Part model, mm, in its own coordinate system. Give positions to 0.01 mm unless a question says otherwise; leave off trailing zeros. Loops run counter-clockwise (first coordinate to the right, second up) from the corner with the lowest first, then second, coordinate; pieces in that order, holes last. Notation, with made-up numbers: M 28.25,78 L 83.25,78 A22 ccw 83.25,86 Z; hole C -24.5,42.25 d6. An arc over 180 degrees is marked long. Put each result on its own line as item: value. Start each with the question number.
```python
from build123d import *

# Parameters (mm, degrees)
BOSS_EXTRU_1_DEPTH = 100
CONG_1_R           = 30


with BuildPart() as part:
    # Esquisse1 → Boss.-Extru.1 (new body)
    with BuildSketch(Plane.XY):
        with BuildLine():
            Line((36.827299657, 30), (22.5, 30))
            ThreePointArc((22.5, 30), (33.541019662, 16.770509831), (37.5, 0))
            ThreePointArc((37.5, 0), (33.541019662, -16.770509831), (22.5, -30))
            Line((22.5, -30), (36.827299657, -30))
            ThreePointArc((36.827299657, -30), (44.752355992, -15.920949505), (47.5, 0))
            ThreePointArc((47.5, 0), (44.752355992, 15.920949505), (36.827299657, 30))
        make_face()
    extrude(amount=BOSS_EXTRU_1_DEPTH)

    # Congé1
    # the kernel refuses this fillet: 30 mm, written as the material it takes off along each edge
    with BuildSketch(Plane(origin=(111.827299657, 30, 100), x_dir=(0, 0, -1), z_dir=(-1, 0, 0))) as cong_1_piece_1:
        with BuildLine():
            CenterArc((CONG_1_R, CONG_1_R), CONG_1_R, 180, 90)
            Line((0, CONG_1_R), (0, 0))
            Line((0, 0), (CONG_1_R, 0))
        make_face()
    extrude(amount=164.327299657, mode=Mode.SUBTRACT)
    with BuildSketch(Plane(origin=(-52.5, -30, 100), x_dir=(0, 1, 0), z_dir=(1, 0, 0))) as cong_1_piece_2:
        with BuildLine():
            CenterArc((CONG_1_R, -CONG_1_R), CONG_1_R, 90, 90)
            Line((0, -CONG_1_R), (0, 0))
            Line((0, 0), (CONG_1_R, 0))
        make_face()
    extrude(amount=164.327299657, mode=Mode.SUBTRACT)


solid = part.part
```
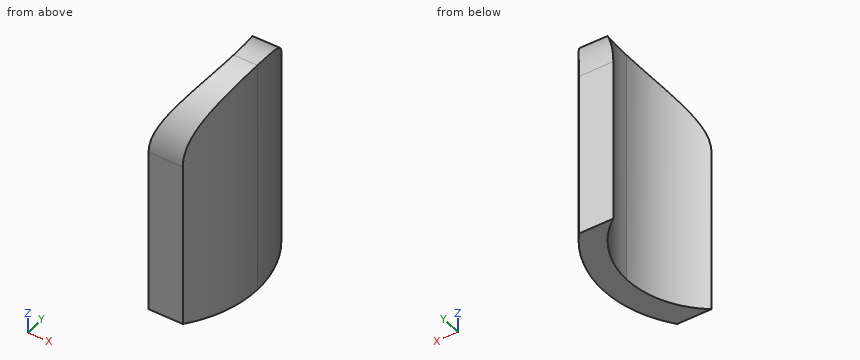
1) Band-saw the part on A-A on x = 32.5. Give the cut face in (y, z), then the cut area to 3 significant figures.
2) Band-saw the part on C-C on y = -15. Give the cut face in (x, z), then the cut area to 3 significant figures.
3) Band-saw the part on D-D on x = 46. Give the cut face in (y, z), then the cut area to 3 significant figures.
4) Pin check, flat tips, straight feed: pin 1 Ø6 at (y, z) = (5.5, 74) entering from +X; pin 2 Ø3 at (x, y) = (38.5, 17.5) entering from +Z; pin 3 Ø8 at (y, z) = (-6.5, 84) entering from -X; pin 4 Ø10 at (x, z) = (41.5, 21.5) entering from -Y. Stop position of each tip, or through.
5) Wall check: L1, parallel to Y at x = 37.75, z = 39; L2, parallel to Z at x = 42.5, y = 0.5; L3, parallel to X at y = -15.5, z = 56.5. Give the ranges that are in metal, low to high.
6) Band-saw the part on B-B on z = 66. Give the cut face in (x, y), then the cut area to 3 significant figures.
Evaluation:
1. outline: M -30,0 L -18.71,0 L -18.71,93.45 A30 ccw -30,70 Z; M 18.71,0 L 30,0 L 30,70 A30 ccw 18.71,93.45 Z
1. area: 1,950 mm2
2. outline: M 34.37,0 L 45.07,0 L 45.07,95.98 L 34.37,95.98 Z
2. area: 1,030 mm2
3. outline: M -11.84,0 L 11.84,0 L 11.84,97.56 A30 ccw -11.84,97.56 Z
3. area: 2,350 mm2
4. pin 1: x = 47.43
4. pin 2: z = 95.38
4. pin 3: x = 36
4. pin 4: y = -30
5. L1: -28.83 to 28.83
5. L2: 0 to 100
5. L3: 34.15 to 44.9
6. outline: M 22.5,-30 L 36.83,-30 A47.5 ccw 36.83,30 L 22.5,30 A37.5 cw Z
6. area: 668 mm2
